from build123d import *

# Parameters (mm, degrees)
HEX_KEY_1_DEPTH     = 4
CHAMFER_HEAD_SIZE   = 0.5
CHAMFER_THREAD_SIZE = 0.5


with BuildPart() as part:
    # Sketch1 → Main Body (revolve)
    with BuildSketch(Plane.XY, mode=Mode.PRIVATE) as main_body_sk:
        with BuildLine():
            Line((5, 42), (9, 42))
            Line((9, 42), (9, 33.398922974))
            Line((9, 33.398922974), (12, 32))
            Line((12, 32), (12, 30))
            Line((12, 30), (6.4, 30))
            ThreePointArc((6.4, 30), (6.117157288, 29.882842712), (6, 29.6))
            Line((6, 29.6), (6, 0))
            Line((6, 0), (0, 0))
            Line((0, 0), (0, 32.995696905))
            Line((0, 32.995696905), (5, 36))
            Line((5, 36), (5, 42))
        make_face()
    revolve(main_body_sk.sketch.rotate(Axis((0, 0, 0), (0, 1, 0)), 90), axis=Axis((0, 0, 0), (0, 1, 0)))  # turned: the seam where the file's is

    # Sketch2 → Hex Key 1 (cut)
    with BuildSketch(Plane(origin=(0, 42, 0), x_dir=(1, 0, 0), z_dir=(0, 1, 0))):
        Polygon((-5.7908232, 0), (-2.8954116, -5.015), (2.8954116, -5.015), (5.7908232, 0), (2.8954116, 5.015), (-2.8954116, 5.015), align=None)
    extrude(amount=-HEX_KEY_1_DEPTH, mode=Mode.SUBTRACT)

    # Chamfer-Head
    chamfer_head_edges = [part.edges().sort_by_distance(p)[0] for p in [
        (0, 42, 9),
    ]]
    chamfer(chamfer_head_edges, length=CHAMFER_HEAD_SIZE)

    # Chamfer-Thread
    chamfer_thread_edges = [part.edges().sort_by_distance(p)[0] for p in [
        (0, 0, 6),
    ]]
    chamfer(chamfer_thread_edges, length=CHAMFER_THREAD_SIZE)


solid = part.part
Source: CAD feature listing. Evaluate the final solid. Frame: model axes, mm. A direction names the side the tool comes from. Give positions to 0.01 mm unless a question says otherwise; leave off trailing zeros. Write each loop counter-clockwise with the first axis right and the second up, starting at its lowest first coordinate (ties: lowest second). Pieces come first, ordered by that corner, then holes. Notation, with made-up numbers: M -7.5,5 L 34.5,5 A30 cw 34.5,40 Z; hole C 57,31 d5. An arc over 180 degrees is marked long. Return JSON: item names as keys, results as strings. Group by question number.
1) Set-up query: faces 1 (the face through (-4.323, 40.028, -2.543)), 2 (the face through (-1.802, 14.846, -5.723)), 3 (the face through (-4, 42, 4)). Return all of +Z, -Z, +X, -X, +Y, -Y with unobstructed straight access to the full face (end or side cutting, diameter ignored); none if empty.
2) First-contact query: pin 1 Ø5 at (x, z) = (2.5, 0.5) entering from +Y; pin 2 Ø3 at (x, z) = (-5, 7) entering from -Y; pin 3 Ø3 at (y, z) = (9.5, 9) entering from +X; pin 4 Ø3 at (x, y) = (-5.5, 18) entering from -Z. Flat tips, straight axial feed; report the tip coordinate or a pass-through.
3) Cut plane A-A, the plane y = 6. Output: boundary loops of the cut face in (x, z).
4) Ray query, L1, parallel to X at y = 37.2, z = 0; L2, parallel to Y at x = -1, z = 7.5; L3, parallel to Z at x = -4.5, y = 39. Return the intervals inside material, ascending.
5) Cut plane B-B, the plane y = 31.5. Output: boundary loops of the cut face in (x, z).
6) Draft query along Z for faces 4 (the face through (8.97, 33.31, 1.99)), 5 (the face through (5, 30, -5)), 6 (the face through (0, 37, 5)). Return one class per face: released by +Z, released by -Z, zero draft, split by the parting line, or undercut.
Data:
{
 "1": {"face 1": "+Y", "face 2": "-Y", "face 3": "+Z, -Z, +X, -X, +Y"},
 "2": {"pin 1": "stops at y = 38", "pin 2": "stops at y = 30", "pin 3": "passes through", "pin 4": "stops at z = -4.47"},
 "3": {"outline": "C 0,0 d12"},
 "4": {"L1": "x = -9 to -5, 5 to 9", "L2": "y = 30 to 42", "L3": "z = -7.79 to -2.24, 2.24 to 7.79"},
 "5": {"outline": "C 0,0 d24"},
 "6": {"face 4": "split by the parting line", "face 5": "zero draft", "face 6": "undercut"}
}
